Work out the finished part from the listing and answer in its coordinate system (mm). A direction names the side the tool comes from. Round coordinates to 2 decimals unless told otherwise and drop trailing zeros. Order: outer loops, then holes, each group sorted by start corner. A loop starts at its lowest first (then second) coordinate and runs counter-clockwise, first axis right, second up. Notation, with made-up numbers: (85, 50) - (90, 50) arc R14 ccw to (90, 72) - close; hole circle Ø6 at (39, -25). An arc over 180 degrees is marked (long way). Put each result on its own line as item: value.
```python
from build123d import *

# Parameters (mm, degrees)
BOSS_EXTRUDE1_DEPTH      = 3
BOSS_EXTRUDE1_DEPTH_BACK = 3
SKETCH1_R                = 1.7
CUT_EXTRUDE1_DEPTH       = 1.35
CUT_EXTRUDE1_DEPTH_BACK  = 1.35
CUT_EXTRUDE1_START       = -3
FILLET1_R                = 2
FILLET2_R                = 0.5
FILLET3_R                = 4
FILLET4_R                = 4
FILLET5_R                = 4
FILLET6_R                = 0.5
FILLET7_R                = 0.5


with BuildPart() as part:
    # Sketch1 → Boss-Extrude1 (new, two sides: drawn at the far end of the back side and taken through both)
    with BuildSketch(Plane.XY.offset(-BOSS_EXTRUDE1_DEPTH_BACK)):
        with BuildLine():
            Line((0, 0), (0, 14.741701813))
            Line((0, 14.741701813), (9, 14.741701813))
            Line((9, 14.741701813), (37.931461615, -51.19641531))
            ThreePointArc((37.931461615, -51.19641531), (36.98891746, -53.791598658), (34.3522375, -52.972278891))
            Line((34.3522375, -52.972278891), (8, -5.601660306))
            Line((8, -5.601660306), (0, 0))
        make_face()
        with Locations((4.1, 8.741701813)):
            Circle(SKETCH1_R, mode=Mode.SUBTRACT)
    extrude(amount=BOSS_EXTRUDE1_DEPTH + BOSS_EXTRUDE1_DEPTH_BACK)

    # Sketch2 → Cut-Extrude1 (cut, two sides: drawn at the far end of the back side and taken through both)
    with BuildSketch(Plane.XY.offset(3).offset(CUT_EXTRUDE1_START - CUT_EXTRUDE1_DEPTH_BACK)):
        Polygon((0, 0), (0, 14.741701813), (8.2, 14.741701813), (8.2, 5.741701813), align=None)
    extrude(amount=CUT_EXTRUDE1_DEPTH + CUT_EXTRUDE1_DEPTH_BACK, mode=Mode.SUBTRACT)

    # Fillet1
    fillet1_edges = [part.edges().sort_by_distance(p)[0] for p in [
        (8.2, 5.741701813, 0),
    ]]
    fillet(fillet1_edges, radius=FILLET1_R)

    # Fillet2
    fillet2_edges = [part.edges().sort_by_distance(p)[0] for p in [
        (0, 0, 0),
    ]]
    fillet(fillet2_edges, radius=FILLET2_R)

    # Fillet3
    fillet3_edges = [part.edges().sort_by_distance(p)[0] for p in [
        (8, -5.601660306, 0),
    ]]
    fillet(fillet3_edges, radius=FILLET3_R)

    # Fillet4
    # the kernel refuses this fillet: 4 mm, written as the material it takes off along each edge
    with BuildSketch(Plane(origin=(9, 14.741701813, 9.532571038), x_dir=(0.4017923449729062, -0.9157308073452443, 0), z_dir=(0, 0, -1))) as fillet4_piece_1:
        with BuildLine():
            CenterArc((FILLET4_R * 0.653257103757, FILLET4_R), FILLET4_R, 203.690274531, 66.309725469)
            Line((-FILLET4_R * 0.262473703589, FILLET4_R * 0.598207655027), (0, 0))
            Line((0, 0), (FILLET4_R * 0.653257103757, 0))
        make_face()
    extrude(amount=19.065142075, mode=Mode.SUBTRACT)

    # Fillet5
    fillet5_edges = [part.edges().sort_by_distance(p)[0] for p in [
        (0, 0, 2.175),
    ]]
    fillet(fillet5_edges, radius=FILLET5_R)

    # Fillet6
    fillet6_edges = [part.edges().sort_by_distance(p)[0] for p in [
        (0, 14.741701813, -2.175),
        (0, 14.741701813, 2.175),
        (8.2, 14.307221126, 0),
    ]]
    fillet(fillet6_edges, radius=FILLET6_R)

    # Fillet7
    fillet7_edges = [part.edges().sort_by_distance(p)[0] for p in [
        (4.475927023, -3.134077842, 3),
        (0.451956667, 0.235273749, 3),
        (4.475927023, -3.134077842, -3),
        (0.451956667, 0.235273749, -3),
        (0, 8.161985008, -3),
        (0.146446609, 14.595255204, -3),
        (0, 8.161985008, 3),
        (0.146446609, 14.595255204, 3),
        (36.98891746, -53.791598658, -3),
        (23.990678215, -19.423772058, -3),
        (36.98891746, -53.791598658, 3),
        (23.990678215, -19.423772058, 3),
        (21.399808273, -29.689072498, 3),
        (21.399808273, -29.689072498, -3),
        (7.922396855, -5.671641436, 3),
        (7.922396855, -5.671641436, -3),
        (3.443485792, 14.741701813, 3),
        (8.574587008, 14.090483496, 3),
        (3.443485792, 14.741701813, -3),
        (8.574587008, 14.090483496, -3),
    ]]
    fillet(fillet7_edges, radius=FILLET7_R)


solid = part.part
```
1) A cutting plane is placed at B-B on x = 4.1. Give the number of separate pieces and of enclosed holes in the cut face, then the cut area to 3 significant figures.
Findings below:
separate pieces: 3
enclosed holes: 0
area: 62.2 mm2
2) Given pin 1 Ø1 at (y, z) = (-22.5, -0.5) entering from +X; pin 2 Ø5.5 at (x, y) = (4.1, 8.74) entering from +Z; pin 3 Ø2 at (x, z) = (17.5, -0.5) entering from +Y; pin 4 Ø3 at (x, z) = (8, 1.5) entering from -Y, each flat-ended and moving along its own axis, determine where each tip first touches the part or whether it passes through.
Findings below:
pin 1: stops at x = 25.56
pin 2: stops at z = 3
pin 3: stops at y = -2.35
pin 4: stops at y = -8.3
3) A cutting plane is placed at A-A on z = -0.25. Write down the section's boundary in (x, y).
Findings below:
outline: (0.44, 0.26) arc R4 ccw to (1.71, -1.19) - (7.25, -5.07) arc R4 cw to (8.45, -6.41) - (34.35, -52.97) arc R2 ccw to (37.93, -51.2) - (10.05, 12.35) arc R4 ccw to (9.03, 13.74) arc R0.5 ccw to (8.2, 13.37) - (8.2, 6.78) arc R2 cw to (7.35, 5.14) - (0.58, 0.41) arc R0.5 ccw to start
4) For faces 1 (the cylindrical face through (21.35, -29.29, -2.86)), 2 (the flat face through (4, 2.8, 0)), determine the directions among +Z, -Z, +X, -X, +Y, -Y from which every point of the face is accessible in a straight line to the end or side of a thin tool.
Findings below:
face 1: -Z, -X, -Y
face 2: -X, +Y
5) Straight lines are drawn through the part: L1, parallel to Y at x = 5.5, z = 1.5; L2, parallel to Y at x = 4.1, z = -1.8; L3, parallel to X at y = -3.5, z = 0.5. For each, find the intervals that lie inside material, in ascending order. Write a range as from..to.
Findings below:
L1: y = -3.85..7.78, 9.71..14.74
L2: y = -2.87..7.04, 10.44..14.74
L3: x = 5..17
6) For a pull along X with two mould halves and no side action, classify faces 3 (the cylindrical face through (3.731, 7.082, 2.163)), 4 (the cylindrical face through (0.68, -0.15, 0.04)), 5 (the cylindrical face through (37.03, -53.77, -0.04)) as pulls with the +X half, pulls with the -X half, needs draft (parallel to the pull), parting line crosses it, or undercut.
Findings below:
face 3: undercut
face 4: pulls with the -X half
face 5: parting line crosses it
